Input: part model. Units: mm. Frame: model coordinates. Face numbers are marked on the shaded views. A direction names the side the tool comes from. Coordinates: 2 decimals unless noted, no trailing zeros. Loops run counter-clockwise (first coordinate to the right, second up) from the corner with the lowest first, then second, coordinate; pieces in that order, holes last.
Item 1: Contact query for flat-ended pins moving along their axis: P1, Ø3, axis at x = -5, z = 2.5, coming from the +Y side; P2, Ø3, axis at y = -20.5, z = 3, coming from the -X side; P3, Ø2.5, axis at x = 0, y = -8.5, coming from the -Z side. Output: stop coordinate, or through.
Item 2: Reachability of the marked faces 1 and 2 from +Z, -Z, +X, -X, +Y, -Y: full face, straight path, thin tool, end or side. Return the list, or none.
Item 3: Section D-D on z = 1.55. Return loops of the section in (x, y), and give its area (3 significant figures).
Item 4: Pull-direction query (Y, two-part tool) for the marked faces 3, 4 and 5; classes: released by +Y, released by -Y, zero draft, split by the parting line, or undercut.
Item 5: Section B-B on z = 5.65. Return loops of the section in (x, y).
Item 6: Section C-C on y = -8.5. Return loops of the section in (x, z).
Item 7: Ray query, line 1 along Y through (x, z) = (0, 5.7); line 2 along Y through (x, z) = (-0.5, 5.2); line 3 along Z through (x, y) = (-2.25, -1). Return the intervals inside material, ascending.
Item 8: Section A-A on x = 0. Return loops of the section in (y, z), and give its area (3 significant figures).
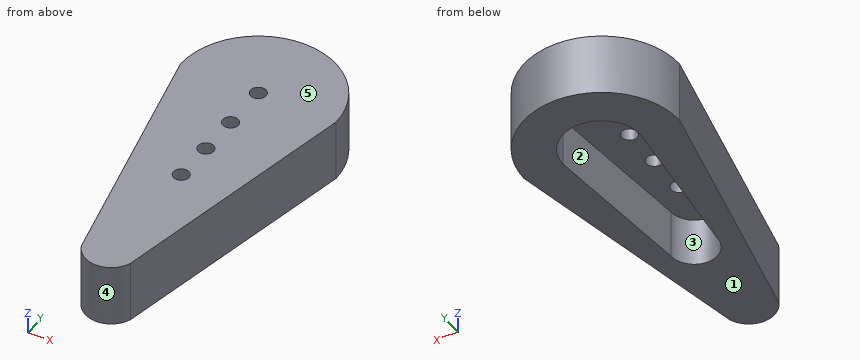
```python
from build123d import *

# Parameters (mm, degrees)
BOSS_EXTRUDE1_DEPTH     = 6
CUT_EXTRUDE3_DEPTH      = 4.7
CUT_EXTRUDE4_DEPTH      = 28.796807371
CUT_EXTRUDE4_DEPTH_BACK = 28.796807371
SKETCH4_R               = 0.75
SKETCH6_R               = 0.75
CUT_EXTRUDE6_DEPTH      = 28.796807371
LPATTERN1_COUNT         = 3
LPATTERN1_PITCH         = 4


with BuildPart() as part:
    # Sketch2 → Boss-Extrude1 (new body)
    with BuildSketch(Plane.XY):
        with BuildLine():
            Line((-7.5, 0), (-2.347339189, -24.710231791))
            ThreePointArc((-2.347339189, -24.710231791), (0.004409749, -26.349996111), (2.350359302, -24.70194551))
            Line((2.350359302, -24.70194551), (7.5, 0))
            ThreePointArc((7.5, 0), (0, 7.5), (-7.5, 0))
        make_face()
    extrude(amount=BOSS_EXTRUDE1_DEPTH)

    # Sketch3 → Cut-Extrude3 (cut)
    with BuildSketch(Plane.XY):
        with BuildLine():
            Line((-3.75, 0), (-2.25, -15))
            ThreePointArc((-2.25, -15), (0, -17.25), (2.25, -15))
            Line((2.25, -15), (3.75, 0))
            ThreePointArc((3.75, 0), (0, 3.75), (-3.75, 0))
        make_face()
    extrude(amount=CUT_EXTRUDE3_DEPTH, mode=Mode.SUBTRACT)

    # Sketch4 → Cut-Extrude4 (cut, two sides: drawn at the far end of the back side and taken through both)
    with BuildSketch(Plane(origin=(0, 0, 4.7), x_dir=(-1, 0, 0), z_dir=(0, 0, -1)).offset(-CUT_EXTRUDE4_DEPTH_BACK)):
        Circle(SKETCH4_R)
    extrude(amount=CUT_EXTRUDE4_DEPTH + CUT_EXTRUDE4_DEPTH_BACK, mode=Mode.SUBTRACT)

    # Sketch6 → Cut-Extrude6 (cut, symmetric)
    with BuildSketch(Plane(origin=(0, 0, 4.7), x_dir=(-1, 0, 0), z_dir=(0, 0, -1))):
        with Locations((0, -4.5)):
            Circle(SKETCH6_R)
    cut_extrude6 = extrude(amount=CUT_EXTRUDE6_DEPTH, both=True, mode=Mode.SUBTRACT)

    # LPattern1: Cut-Extrude6 ×3
    with Locations(*[(0, -i * LPATTERN1_PITCH, 0) for i in range(1, LPATTERN1_COUNT)]):
        add(cut_extrude6, mode=Mode.SUBTRACT)


solid = part.part
```
Results found:
1. P1: stops at y = 6.63
1. P2: stops at x = -3.54
1. P3: stops at z = 4.7
2. face 1: -Z, +X, -X, +Y, -Y
2. face 2: -Z
3. outline: (-7.5, 0) - (-2.35, -24.71) arc R2.5 ccw to (2.35, -24.7) - (7.5, 0) arc R7.5 ccw to start; hole (-3.75, 0) - (-2.25, -15) arc R2.25 ccw to (2.25, -15) - (3.75, 0) arc R3.75 ccw to start
3. area: 217 mm2
4. face 3: undercut
4. face 4: released by -Y
4. face 5: zero draft
5. outline: (-7.5, 0) - (-2.35, -24.71) arc R2.5 ccw to (2.35, -24.7) - (7.5, 0) arc R7.5 ccw to start; hole circle Ø1.5 at (0, -12.5); hole circle Ø1.5 at (0, -8.5); hole circle Ø1.5 at (0, -4.5); hole circle Ø1.5 at (0, 0)
6. outline: (-5.73, 0) - (-2.9, 0) - (-2.9, 4.7) - (-0.75, 4.7) - (-0.75, 6) - (-5.73, 6) - close; (0.75, 4.7) - (2.9, 4.7) - (2.9, 0) - (5.73, 0) - (5.73, 6) - (0.75, 6) - close
7. line 1: y = -26.35 to -13.25, -11.75 to -9.25, -7.75 to -5.25, -3.75 to -0.75, 0.75 to 7.5
7. line 2: y = -26.3 to -13.06, -11.94 to -9.06, -7.94 to -5.06, -3.94 to -0.56, 0.56 to 7.48
7. line 3: z = 4.7 to 6
8. outline: (-26.35, 0) - (-17.25, 0) - (-17.25, 4.7) - (-13.25, 4.7) - (-13.25, 6) - (-26.35, 6) - close; (-11.75, 4.7) - (-9.25, 4.7) - (-9.25, 6) - (-11.75, 6) - close; (-7.75, 4.7) - (-5.25, 4.7) - (-5.25, 6) - (-7.75, 6) - close; (-3.75, 4.7) - (-0.75, 4.7) - (-0.75, 6) - (-3.75, 6) - close; (0.75, 4.7) - (3.75, 4.7) - (3.75, 0) - (7.5, 0) - (7.5, 6) - (0.75, 6) - close
8. area: 96.6 mm2
